```python
from build123d import *

# Parameters (mm, degrees)
SKETCH_1_W          = 550
SKETCH_1_H          = 122
EXTRUDE_1_DEPTH     = 3
CUT_EXTRUDE_2_DEPTH = 282.700195243
SKETCH_2_R          = 3
SKETCH_2_R_2        = 2
CUT_EXTRUDE_1_DEPTH = 10
CHAMFER_1_SIZE      = 2


with BuildPart() as part:
    # 草图1 → 凸台-拉伸1 (new body)
    with BuildSketch(Plane.XY):
        Rectangle(SKETCH_1_W, SKETCH_1_H)
    extrude(amount=EXTRUDE_1_DEPTH)

    # 草图3 → 切除-拉伸2 (cut, through all)
    with BuildSketch(Plane.XY.offset(3)):
        Polygon((-275, 31), (-245, 31), (-245, -31), (-227.679491924, -61), (-275, -61), align=None)
        Polygon((245, -31), (227.679491924, -61), (275, -61), (275, 31), (245, 31), align=None)
    extrude(amount=-CUT_EXTRUDE_2_DEPTH, mode=Mode.SUBTRACT)

    # 草图2 → 切除-拉伸1 (cut)
    with BuildSketch(Plane.XY):
        with Locations((-200, 42.5)):
            Circle(SKETCH_2_R)
        with Locations((-234, 42.5)):
            Circle(SKETCH_2_R)
        with Locations(Location((234, 42.5, 0), (0, 0, 180))):
            Circle(SKETCH_2_R)
        with Locations(Location((200, 42.5, 0), (0, 0, 180))):
            Circle(SKETCH_2_R)
        with Locations((-265, 46)):
            Circle(SKETCH_2_R_2)
        with Locations((-100, 46)):
            Circle(SKETCH_2_R_2)
        with Locations((-225, -46)):
            Circle(SKETCH_2_R_2)
        with Locations((-70, -46)):
            Circle(SKETCH_2_R_2)
        with Locations(Location((225, -46, 0), (0, 0, 180))):
            Circle(SKETCH_2_R_2)
        with Locations(Location((70, -46, 0), (0, 0, 180))):
            Circle(SKETCH_2_R_2)
        with Locations(Location((100, 46, 0), (0, 0, 180))):
            Circle(SKETCH_2_R_2)
        with Locations(Location((265, 46, 0), (0, 0, 180))):
            Circle(SKETCH_2_R_2)
    extrude(amount=CUT_EXTRUDE_1_DEPTH, mode=Mode.SUBTRACT)

    # 倒角1
    chamfer_1_edges = [part.edges().sort_by_distance(p)[0] for p in [
        (227, -46, 3),
        (-72, -46, 3),
        (-227, -46, 3),
        (-102, 46, 3),
        (-267, 46, 3),
        (72, -46, 3),
        (102, 46, 3),
        (267, 46, 3),
    ]]
    chamfer(chamfer_1_edges, length=CHAMFER_1_SIZE)


solid = part.part
```
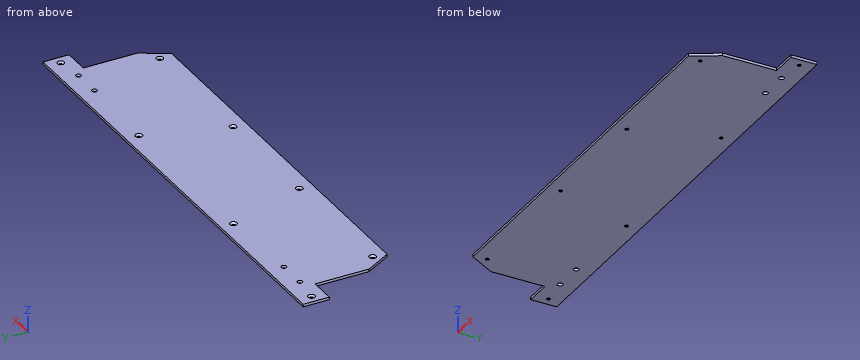
Part model, mm, in its own coordinate system. Coordinates: 2 decimals unless noted, no trailing zeros. Loops run counter-clockwise (first coordinate to the right, second up) from the corner with the lowest first, then second, coordinate; pieces in that order, holes last. Notation, with made-up numbers: (-24, -34.75) - (-9, -34.75) arc R23 cw to (-9, -9.75) - close; hole circle Ø10 at (69, -29). An arc over 180 degrees is marked (long way). Write item = value, one per line. Start each with the question number.
Item 1: Cut at A-A, the plane z = 2.3. State how many separate pieces and enclosed holes the cut face has, and give its area (3 significant figures).
Item 2: Cut at B-B, the plane y = -36. Give the cut face in (x, z), and give its area (3 significant figures).
Item 3: Flat gauge pins, fed straight in: pin 1 Ø2.5 at (x, y) = (100, 46) entering from +Z; pin 2 Ø1.5 at (x, z) = (-260.5, 1.5) entering from -Y; pin 3 Ø0.9 at (y, z) = (3.5, 2) entering from +X; pin 4 Ø4.5 at (x, y) = (-265, 46) entering from +Z. Where does each tip first touch, or does it go through?
Item 4: Wall check: L1, parallel to Y at x = -200, z = 0.9; L2, parallel to X at y = 42.5, z = 1.65; L3, parallel to X at y = -46, z = 0.2. Give the ranges that are in metal, low to high. Write a range as from..to.
The answers:
q1.separate_pieces = 1
q1.enclosed_holes = 12
q1.area = 60,700 mm2
q2.outline = (-242.11, 0) - (242.11, 0) - (242.11, 3) - (-242.11, 3) - close
q2.area = 1,450 mm2
q3.pin_1 = through
q3.pin_2 = 31
q3.pin_3 = 245
q3.pin_4 = 1.25
q4.L1 = -61..39.5, 45.5..61
q4.L2 = -275..-237, -231..-203, -197..197, 203..231, 237..275
q4.L3 = -236.34..-227, -223..-72, -68..68, 72..223, 227..236.34
